```python
from build123d import *

# Parameters (mm, degrees)
F0_W     = 76.2
F0_H     = 76.2
F1_DEPTH = 19.05
F3_D     = 9.525
F4_R     = 6.35
F5_R     = 4.445


with BuildPart() as f1:
    # F0 (on Top) → F1 (new body)
    with BuildSketch(Plane.XY):
        Rectangle(F0_W, F0_H)
    extrude(amount=F1_DEPTH)

    # F3 (through all)
    with Locations(Plane(origin=(-38.1, 0, 0), x_dir=(0, -1, 0), z_dir=(-1, 0, 0))):
        with Locations((-25.4, 9.525), (25.4, 9.525)):
            Hole(F3_D / 2)

    # F4
    f4_edges = [f1.edges().sort_by_distance(p)[0] for p in [
        (0, -38.1, 19.05),
        (0, -38.1, 0),
        (0, 38.1, 19.05),
        (0, 38.1, 0),
    ]]
    fillet(f4_edges, radius=F4_R)

    # F5
    f5_edges = [f1.edges().sort_by_distance(p)[0] for p in [
        (-38.1, 0, 19.05),
        (38.1, 0, 19.05),
    ]]
    fillet(f5_edges, radius=F5_R)


solid = f1.part
```
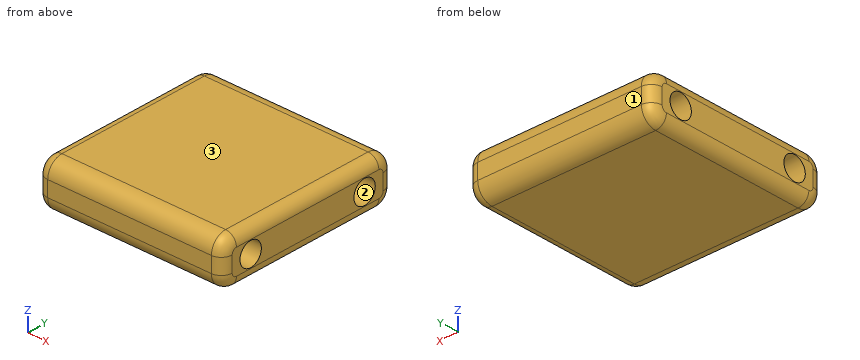
Can you work these out from the model? Positions are in its coordinate system, mm. Face numbers are marked on the shaded views. Coordinates: 2 decimals unless noted, no trailing zeros. Write each loop counter-clockwise with the first axis right and the second up, starting at its lowest first coordinate (ties: lowest second). Pieces come first, ordered by that corner, then holes. Notation, with made-up numbers: M 71.5,8 L 93.5,8 A25 cw 93.5,41 Z; hole C 44,33 d3. An arc over 180 degrees is marked long. Answer as CSV lines item,"result".
Item 1: Please list where these lines run through material, in increasing order: line 1 along Z through (x, y) = (-21, 25.4); line 2 along Y through (x, z) = (24.5, 7.5); line 3 along Y through (x, z) = (-18.5, 13).
Geometry results:
line 1,"z = 0 to 4.76, 14.29 to 19.05"
line 2,"y = -38.1 to -29.71, -21.09 to 21.09, 29.71 to 38.1"
line 3,"y = -38.09 to -28.66, -22.14 to 22.14, 28.66 to 38.09"
Item 2: I'm going to push flat-ended pins straight in: P1, Ø1.5, axis at y = -18.5, z = 16, coming from the +X side; P2, Ø7.5, axis at y = -25.4, z = 9.525, coming from the +X side. Where does each tip first touch, or does it pass through?
Geometry results:
P1,"stops at x = 38.05"
P2,"passes through"
Item 3: Imagine slicing it at C-C on y = 25. List the corners of the cut face in (x, z) for me (3 decimals), plus the area to 3 significant figures.
Geometry results:
outline,"M -38.1,4.445 A4.445 ccw -33.655,0 L 33.655,0 A4.445 ccw 38.1,4.445 L 38.1,4.779 L -38.1,4.779 Z; M -38.1,14.271 L 38.1,14.271 L 38.1,14.605 A4.445 ccw 33.655,19.05 L -33.655,19.05 A4.445 ccw -38.1,14.605 Z"
area,"711 mm2"
Item 4: We'd pull the mould along Y, two halves only. Please class the marked faces 1, 2 and 3: +Y half, -Y half, draft (parallel to the pull), parting line (faces both ways), or undercut.
Geometry results:
face 1,"+Y half"
face 2,"undercut"
face 3,"draft"
Item 5: Imagine slicing it at B-B on x = 0. State how many separate pieces and enclosed holes the cut face has, plus the area to 3 significant figures.
Geometry results:
separate pieces,"1"
enclosed holes,"2"
area,"1,270 mm2"
